Work out the finished part from the listing and answer in its coordinate system (mm). A direction names the side the tool comes from. Coordinates: 2 decimals unless noted, no trailing zeros. Write each loop counter-clockwise with the first axis right and the second up, starting at its lowest first coordinate (ties: lowest second). Pieces come first, ordered by that corner, then holes. Notation, with made-up numbers: (68.25, -1.5) - (88.25, -1.5) arc R25 cw to (88.25, 10.5) - close; hole circle Ø1 at (-20, -10.75). An arc over 180 degrees is marked (long way). Use a Markdown table: item, result. Add a question column.
(1) Given pin 1 Ø1.9 at (y, z) = (1, -0.5) entering from -X; pin 2 Ø1.5 at (y, z) = (1.5, -1.5) entering from +X, each flat-ended and moving along its own axis, determine where each tip first touches the part or whether it passes through.
(2) A tool of negligible diameter and unlimited length cuts with its end or side. For faces 5 (the face through (-3.131, -5.525, -0.044)), 6 (the face through (-2.3, -6.2, 3.175)), from which of +Z, -Z, +X, -X, +Y, -Y can it reach the whole face along a straight path? Write none if from no direction.
(3) For a pull along X with two mould halves and no side action, classify faces 1 (the face through (3.131, 5.525, 0.044)), 2 (the face through (-7.559, 5.796, -0.044)), 3 (the face through (6.35, 0, 0)), 4 (the face through (-2.3, -6.2, -3.175)) as released by +X, released by -X, zero draft, split by the parting line, or undercut.
(4) The part is cut by section C-C, the plane x = 3.5. Give the vertices of the cut face in (y, z) (3 decimals).
(5) The part is cut by section A-A, the plane y = 0. Give the vertices of the cut face in (x, z) (3 decimals).
(6) Find the intervals of material crossed by line 1 (X direction, y = -0.25, z = -2.5); line 2 (X direction, y = 3.75, z = -2); line 3 (Y direction, x = -6.25, z = 1.75), in increasing order. Write a range as from..to.
(7) The part is cut by section B-B, the plane z = -2.5. Give the vertices of the cut face in (x, y) (3 decimals).
Autodesk Inventor part; units mm, degrees
ref_plane "YZ Plane" through (0, 0, 0) normal (1, 0, 0) x (0, 1, 0)
ref_plane "XZ Plane" through (0, 0, 0) normal (0, 1, 0) x (-1, 0, 0)
ref_plane "XY Plane" through (0, 0, 0) normal (0, 0, 1) x (1, 0, 0)
sketch "Sketch1" plane through (0, 0, 0) normal (0, 0, 1) x (1, 0, 0)
  circle A0 centre (0, 0) radius 9.525
  line L0 (0, -7.3323) -> (-6.35, -3.6662)
  line L1 (-6.35, -3.6662) -> (-6.35, 3.6662)
  line L2 (-6.35, 3.6662) -> (0, 7.3323)
  line L3 (0, 7.3323) -> (6.35, 3.6662)
  line L4 (6.35, 3.6662) -> (6.35, -3.6662)
  line L5 (6.35, -3.6662) -> (0, -7.3323)
  dimension "d0" = 19.05
  dimension "d1" = 12.7
extrude "Extrusion1" add sketch "Sketch1" along normal mid plane 6.35
properties part number "500 Hex Spacer 0.25" material "Acetal Resin, Black"
Model answer:
| question | item | result |
|---|---|---|
| 1 | pin 1 | x = -9.52 |
| 1 | pin 2 | x = 9.5 |
| 2 | face 5 | +Z, -Z |
| 2 | face 6 | +Z, +X, -X, +Y, -Y |
| 3 | face 1 | undercut |
| 3 | face 2 | split by the parting line |
| 3 | face 3 | undercut |
| 3 | face 4 | zero draft |
| 4 | outline | (-8.859, -3.175) - (-5.312, -3.175) - (-5.312, 3.175) - (-8.859, 3.175) - close; (5.312, -3.175) - (8.859, -3.175) - (8.859, 3.175) - (5.312, 3.175) - close |
| 5 | outline | (-9.525, -3.175) - (-6.35, -3.175) - (-6.35, 3.175) - (-9.525, 3.175) - close; (6.35, -3.175) - (9.525, -3.175) - (9.525, 3.175) - (6.35, 3.175) - close |
| 6 | line 1 | -9.52..-6.35, 6.35..9.52 |
| 6 | line 2 | -8.76..-6.2, 6.2..8.76 |
| 6 | line 3 | -7.19..-3.72, 3.72..7.19 |
| 7 | outline | circle Ø19.05 at (0, 0); hole (-6.35, -3.666) - (0, -7.332) - (6.35, -3.666) - (6.35, 3.666) - (0, 7.332) - (-6.35, 3.666) - close |
